Autodesk Inventor part; units mm, degrees
ref_plane "РабПлоскость2" through (0, 0, 60) normal (0, 0, -1) x (-1, 0, 0)
ref_plane "YZ Plane" through (0, 0, 0) normal (1, 0, 0) x (0, 1, 0)
ref_plane "XZ Plane" through (0, 0, 0) normal (0, 1, 0) x (-1, 0, 0)
sketch "Эскиз1" plane through (0, 0, 0) normal (0, 0, 1) x (1, 0, 0)
  circle A0 centre (0, 0) radius 80
  circle A1 centre (0, 0) radius 90
  line L0 (-90, 0) -> (90, 0)
  point P0 (-80, 0)
  point P1 (80, 0)
  dimension "d0" = 160
  dimension "d1" = 180
extrude "Выдавливание1" add sketch "Эскиз1" along normal blind 120 contours L0 A1 A0 picked at (54.1763, -63.1025)
sketch "Эскиз3" plane through (0, 0, 120) normal (0, 0, 1) x (1, 0, 0)
  arc A0 (-90, 0) -> (90, 0) centre (0, 0) ccw
  line L0 (90, 0) -> (80, 0)
  arc A1 (-80, 0) -> (80, 0) centre (0, 0) ccw
  line L1 (-80, 0) -> (-90, 0)
  circle A2 centre (0, 0) radius 100
  arc A3 (-90, 0) -> (90, 0) centre (0, 0) ccw
  line L2 (-90, 0) -> (-100, 0)
  line L3 (90, 0) -> (100, 0)
  dimension "d7" = 200
extrude "Выдавливание3" add sketch "Эскиз3" along normal blind 5 contours L1 A1 L0 A0 | A0 L3 A2 L2
ref_plane "РабПлоскость2" through (0, 0, 60) normal (0, 0, -1) x (-1, 0, 0)
mirror "Зеркальное отражение1" about plane through (0, 0, 60) normal (0, 0, -1) of "Выдавливание3"
properties part number "Верхняя часть коренного подшипника" material "Бронза, литейная"
Model file for the job. Use its own axes, mm. A direction names the side the tool comes from. Give positions to 0.01 mm unless a question says otherwise; leave off trailing zeros. Loops run counter-clockwise (first coordinate to the right, second up) from the corner with the lowest first, then second, coordinate; pieces in that order, holes last. Notation, with made-up numbers: (12.25, 57) - (37.25, 57) arc R29 cw to (37.25, 89) - close; hole circle Ø8 at (89.25, -7). An arc over 180 degrees is marked (long way). Use one line per item in the form item = value.
(1) Cut at A-A (y = -67.5). Give the cut face in (x, z), then the cut area to 3 significant figures.
Determined:
outline = (-73.78, -5) - (-42.94, -5) - (-42.94, 125) - (-73.78, 125) - (-73.78, 120) - (-59.53, 120) - (-59.53, 0) - (-73.78, 0) - close; (42.94, -5) - (73.78, -5) - (73.78, 0) - (59.53, 0) - (59.53, 120) - (73.78, 120) - (73.78, 125) - (42.94, 125) - close
area = 4,600 mm^2
(2) 3-axis set-ups, long thin cutter, end or side, ignore diameter. For faces 5 (the face through (1.98, -89.98, 59.16)), 6 (the face through (-2.199, -99.976, -2.465)): which of +Z, -Z, +X, -X, +Y, -Y reach the whole face in a straight line?
Determined:
face_5 = -Y
face_6 = +Z, -Z, -Y
(3) Cut at B-B (x = 0). Give the cut face in (y, z).
Determined:
outline = (-100, -5) - (-80, -5) - (-80, 125) - (-100, 125) - (-100, 120) - (-90, 120) - (-90, 0) - (-100, 0) - close
(4) Pull direction Z, two halves, no side cores. Call faces 1 (the face through (-8, -91, 120)), 2 (the face through (-86, 0, 59)), 3 (the face through (0, -83, 125)), 4 (the face through (8, -91, 0)): pulls with the +Z half, pulls with the -Z half, needs draft (parallel to the pull), parting line crosses it, or undercut.
Determined:
face_1 = undercut
face_2 = needs draft
face_3 = pulls with the +Z half
face_4 = undercut
(5) Cut at C-C (y = -85). Give the cut face in (x, z), then the cut area to 3 significant figures.
Determined:
outline = (-52.68, -5) - (52.68, -5) - (52.68, 0) - (29.58, 0) - (29.58, 120) - (52.68, 120) - (52.68, 125) - (-52.68, 125) - (-52.68, 120) - (-29.58, 120) - (-29.58, 0) - (-52.68, 0) - close
area = 8,150 mm^2
(6) Drill centre lines: L1, parallel to Z at x = 21, y = -92.5; L2, parallel to X at y = -60.5, z = 67; L3, parallel to X at y = -61.5, z = 35.5. Where is each one in solid material? Low to high.
Determined:
L1 = -5 to 0, 120 to 125
L2 = -66.63 to -52.34, 52.34 to 66.63
L3 = -65.71 to -51.16, 51.16 to 65.71
(7) Drop flat-ended pins along their axis: P1, Ø3, axis at y = -53, z = 74.5, coming from the +X side; P2, Ø12, axis at x = 33, z = 111, coming from the -Y side; P3, Ø6, axis at y = -58, z = 21, coming from the +X side; P4, Ø12, axis at x = -17.5, y = -76, coming from the -Z side. Give the stop position or say it passes through.
Determined:
P1 = 73.81
P2 = -85.85
P3 = 71.24
P4 = -5
(8) Cut at D-D (z = 38). Give the cut face in (x, y), then the cut area to 3 significant figures.
Determined:
outline = (-90, 0) arc R90 ccw to (90, 0) - (80, 0) arc R80 cw to (-80, 0) - close
area = 2,670 mm^2
